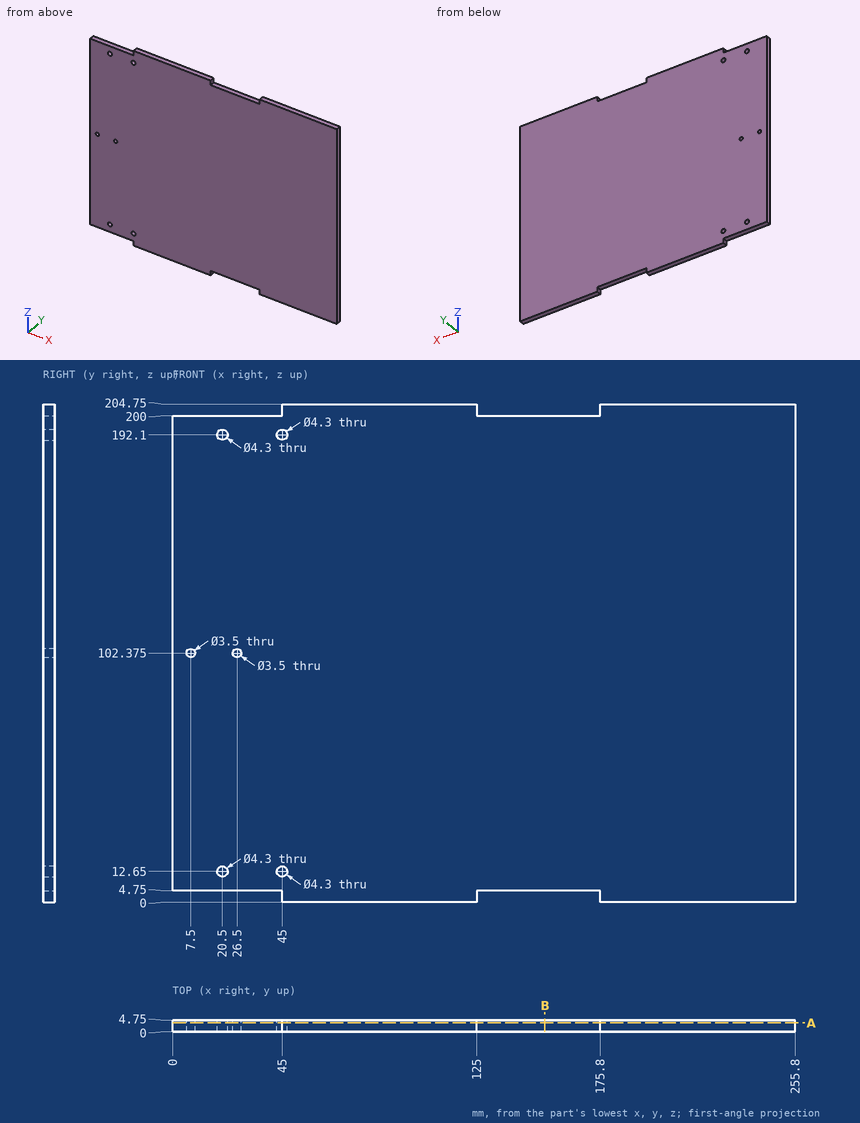
Can you work these out from the drawing? Everything is in mm from the part's minimum corner. Give positions to 0.01 mm unless a question says otherwise; leave off trailing zeros. Order: outer loops, then holes, each group sorted by start corner. A loop starts at its lowest first (then second) coordinate and runs counter-clockwise, first axis right, second up.
Item 1: If we section it at B-B, the plane x = 153: Write out the boundary of the cut face in (y, z).
Item 2: I need wall thicknesses on line 1 (X direction, y = 2.85, z = 192.1); line 2 (Z direction, x = 44.5, y = 4.5); line 3 (Z direction, x = 36, y = 2.05). Which ranges of each line are inside material? Lowest first, please.
Item 3: I'm going to push flat-ended pins straight in: pin 1 (1.4 mm diameter, centred on x = 20.5, y = 3, fed in from +Z); pin 2 (5 mm diameter, centred on x = 20.5, z = 12.65, fed in from -Y); pin 3 (1.4 mm diameter, centred on y = 1.5, z = 203.5, fed in from -X). Where does each tip first touch, or does it pass through?
Item 4: If we section it at A-A, the plane y = 3.7: Write out the boundary of the cut face in (x, z) (3 decimals), plus the area to 3 significant figures.
Values:
1. outline: (0, 4.75) - (4.75, 4.75) - (4.75, 200) - (0, 200) - close
2. line 1: x = 0 to 18.35, 22.65 to 42.85, 47.15 to 255.8
2. line 2: z = 4.75 to 10.56, 14.74 to 190.01, 194.19 to 200
2. line 3: z = 4.75 to 200
3. pin 1: stops at z = 200
3. pin 2: stops at y = 0
3. pin 3: stops at x = 45
4. outline: (0, 4.75) - (45, 4.75) - (45, 0) - (125, 0) - (125, 4.75) - (175.8, 4.75) - (175.8, 0) - (255.8, 0) - (255.8, 204.75) - (175.8, 204.75) - (175.8, 200) - (125, 200) - (125, 204.75) - (45, 204.75) - (45, 200) - (0, 200) - close; hole circle Ø3.5 at (7.5, 102.375); hole circle Ø4.3 at (20.5, 12.65); hole circle Ø4.3 at (20.5, 192.1); hole circle Ø3.5 at (26.5, 102.375); hole circle Ø4.3 at (45, 12.65); hole circle Ø4.3 at (45, 192.1)
4. area: 51,400 mm2
